from build123d import *

# Parameters (mm, degrees)
F1_DEPTH = 140
F2_R     = 10


with BuildPart() as f1:
    # F0 (on Top) → F1 (new body)
    with BuildSketch(Plane.XY):
        with BuildLine():
            ThreePointArc((1.466285, 11.237624), (3.89353, 3.380946), (11.389404, 0))
            Line((11.389404, 0), (88.610596, 0))
            ThreePointArc((88.610596, 0), (96.10647, 3.380946), (98.533715, 11.237624))
            ThreePointArc((98.533715, 11.237624), (90.845598, 135), (98.533715, 258.762376))
            ThreePointArc((98.533715, 258.762376), (96.10647, 266.619054), (88.610596, 270))
            Line((88.610596, 270), (11.389404, 270))
            ThreePointArc((11.389404, 270), (3.89353, 266.619054), (1.466285, 258.762376))
            ThreePointArc((1.466285, 258.762376), (9.154402, 135), (1.466285, 11.237624))
        make_face()
    extrude(amount=F1_DEPTH)

    # F2
    f2_edges = [f1.edges().sort_by_distance(p)[0] for p in [
        (9.154402, 135, 140),
        (3.89353, 3.380946, 140),
        (50, 0, 140),
        (96.10647, 3.380946, 140),
        (90.845598, 135, 140),
        (96.10647, 266.619054, 140),
        (50, 270, 140),
        (3.89353, 266.619054, 140),
    ]]
    fillet(f2_edges, radius=F2_R)


solid = f1.part
Geometry check sheet. Reference: the model listing, model coordinates, mm. Round coordinates to 2 decimals unless told otherwise and drop trailing zeros. Loops run counter-clockwise (first coordinate to the right, second up) from the corner with the lowest first, then second, coordinate; pieces in that order, holes last.
Item 1: Gauge pin test, flat end, axial feed: pin 1 (5 mm diameter, centred on x = 11.5, y = 163, fed in from +Z). Record the tip position at first contact, or that the pin passes through.
Item 2: Mould release check, pull along Y, two halves, no side actions. Record for faces 1 (the cylindrical face through (90.847, 133.263, 64.09)), 2 (the flat face through (49, 137, 0)), 3 (the flat face through (49, 0, 64)): pulls with the +Y half, pulls with the -Y half, needs draft (parallel to the pull), parting line crosses it, or undercut.
Item 3: Thickness scan on line 1 (Z direction, x = 18, y = 91.5); line 2 (X direction, y = 46.5, z = 106); line 3 (X direction, y = 55, z = 14.5). Record the ranges inside material, lowest first.
Item 4: Cross-section at A-A on z = 43. Record the boundary of the cut face in (x, y), then the cut area to 3 significant figures.
Answer sheet:
1. pin 1: stops at z = 138.79
2. face 1: undercut
2. face 2: needs draft
2. face 3: pulls with the -Y half
3. line 1: z = 0 to 140
3. line 2: x = 5.23 to 94.77
3. line 3: x = 5.95 to 94.05
4. outline: (1.47, 11.24) arc R10 ccw to (11.39, 0) - (88.61, 0) arc R10 ccw to (98.53, 11.24) arc R1000 cw to (98.53, 258.76) arc R10 ccw to (88.61, 270) - (11.39, 270) arc R10 ccw to (1.47, 258.76) arc R1000 cw to start
4. area: 23,600 mm2
